For this review, use the dimensioned drawing (mm, ordinates from the lowest corner) and the shaded views. A direction names the side the tool comes from. Give positions to 0.01 mm unless a question says otherwise; leave off trailing zeros. Loops run counter-clockwise (first coordinate to the right, second up) from the corner with the lowest first, then second, coordinate; pieces in that order, holes last. Notation, with made-up numbers: M 29.5,84.25 L 55.5,84.25 A19 cw 55.5,104.25 Z; hole C -4.75,69 d11. An arc over 180 degrees is marked long. Use one line per item in the form item = value. Start each with the question number.
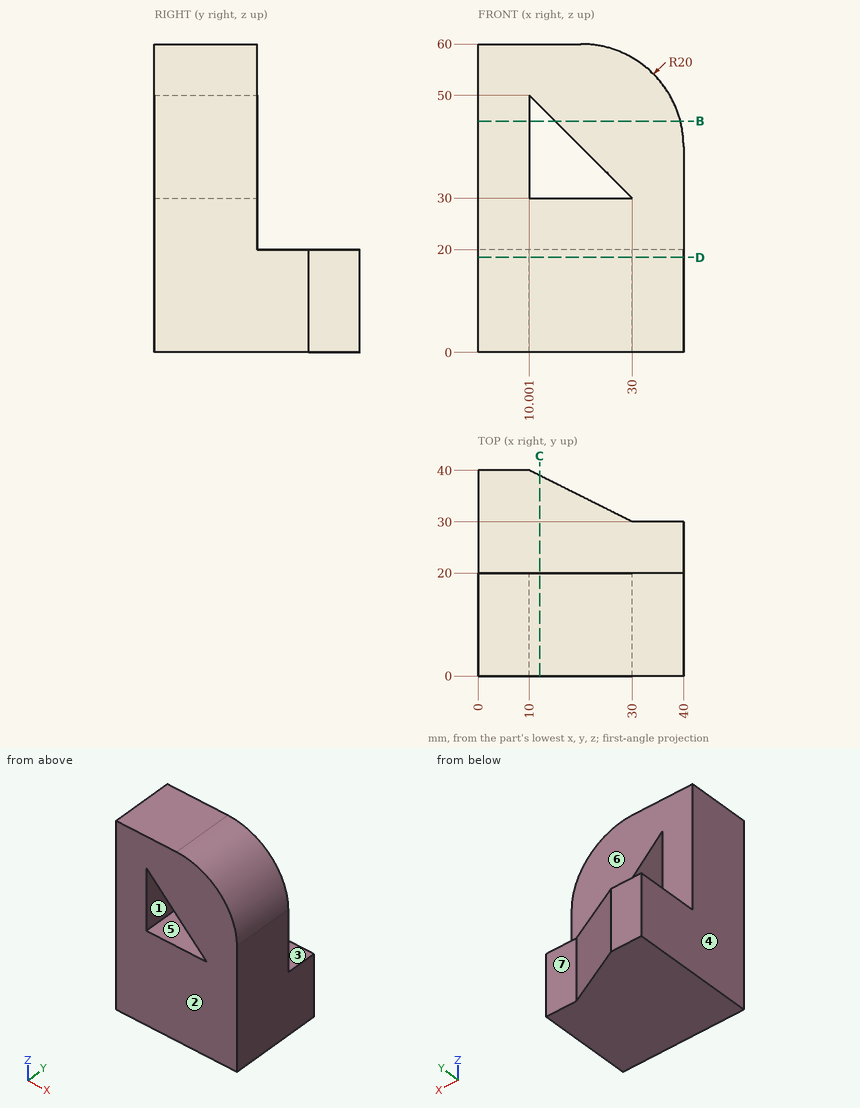
Q1. Take a section at C-C on x = 12. Give the boundary of the cut face in (y, z).
Q2. Clearance check with flat-ended pins moving along their axes: pin 1 Ø8 at (x, z) = (34.5, 13) entering from +Y; pin 2 Ø5 at (y, z) = (33, 8) entering from +X; pin 3 Ø10 at (x, y) = (19, 30) entering from +Z. State where each tip first meets the part, or that it passes through.
Q3. The part is to be moulded in two halves that separate along Z. For the marked faces 1, 2 and 3, say which applies: pulls with the +Z half, pulls with the -Z half, needs draft (parallel to the pull), parting line crosses it, or undercut.
Q4. For the marked faces 4, 5, 6 and 7, list the 3-axis set-ups (+Z, -Z, +X, -X, +Y, -Y) from which the entire face can be reached by the end or side of a thin tool; tool diameter is ignored.
Q5. Wall thickness on probe 1 along X at (y, z) = (9.5, 40); probe 2 along Y at (x, z) = (33, 32.5): over which ranges is each line inside the solid? List them lowest first.
Q6. Take a section at B-B on z = 45. Give the boundary of the cut face in (x, y) (1 decimal), plus the area to 3 significant figures.
Q7. Take a section at D-D on z = 18.5. Give the boundary of the cut face in (x, y).
Response values:
q1.outline = M 0,0 L 39,0 L 39,20 L 20,20 L 20,30 L 0,30 Z; M 0,48 L 20,48 L 20,60 L 0,60 Z
q2.pin_1 = 30
q2.pin_2 = 29
q2.pin_3 = 20
q3.face_1 = undercut
q3.face_2 = needs draft
q3.face_3 = pulls with the +Z half
q4.face_4 = +Z, -Z, -X, +Y, -Y
q4.face_5 = +Y, -Y
q4.face_6 = +Z, +X, -X, +Y
q4.face_7 = +Z, -Z, +X, +Y
q5.probe_1 = 0 to 10, 20 to 40
q5.probe_2 = 0 to 20
q6.outline = M 0,0 L 10,0 L 10,20 L 0,20 Z; M 15,0 L 39.4,0 L 39.4,20 L 15,20 Z
q6.area = 687 mm^2
q7.outline = M 0,0 L 40,0 L 40,30 L 30,30 L 10,40 L 0,40 Z
